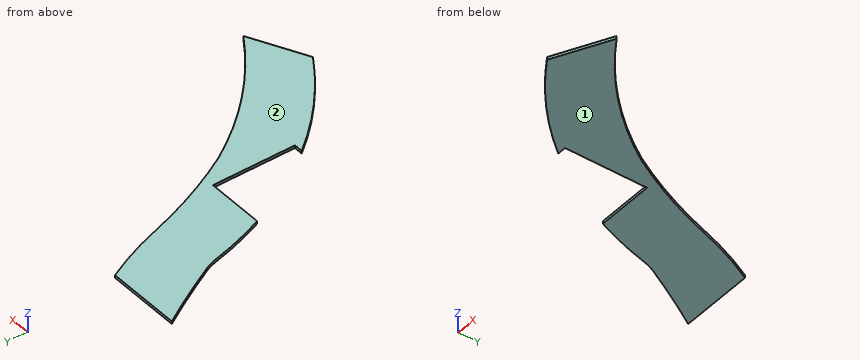
from build123d import *

# Parameters (mm, degrees)
SALIENTE_EXTRUIR1_DEPTH = 0.1


with BuildPart() as part:
    # Model → Saliente-Extruir1 (new body)
    with BuildSketch(Plane.XY):
        with BuildLine():
            Line((34.649371272, 11.960982991), (32.649371272, 10.960982991))
            ThreePointArc((32.649371272, 10.960982991), (30.912697203, 12.270631548), (29.428783982, 13.860982991))
            Line((29.428783982, 13.860982991), (29.750628728, 13.860982991))
            Line((29.750628728, 13.860982991), (29.750628728, 16.860982991))
            Line((29.750628728, 16.860982991), (27.658106466, 16.860982991))
            ThreePointArc((27.658106466, 16.860982991), (27.286967067, 17.858065763), (26.999339741, 18.882365051))
            ThreePointArc((26.999339741, 18.882365051), (26.927371, 19.119642667), (26.826595189, 19.346191565))
            ThreePointArc((26.826595189, 19.346191565), (26.1936862, 20.505212953), (25.516639133, 21.639017009))
            Line((25.516639133, 21.639017009), (28.203922027, 21.639017009))
            ThreePointArc((28.203922027, 21.639017009), (28.714965722, 20.556705993), (29.121100427, 19.430820834))
            ThreePointArc((29.121100427, 19.430820834), (29.792213257, 17.653647808), (30.650628728, 15.958991716))
            ThreePointArc((30.650628728, 15.958991716), (32.427042415, 13.736988846), (34.649371272, 11.960982991))
        make_face()
    extrude(amount=SALIENTE_EXTRUIR1_DEPTH)


solid = part.part
Design review of the part built by this model. Coordinates are the model's own, in mm. Face numbers are marked on the shaded views. Give positions to 0.01 mm unless a question says otherwise; leave off trailing zeros. Loops run counter-clockwise (first coordinate to the right, second up) from the corner with the lowest first, then second, coordinate; pieces in that order, holes last. Notation, with made-up numbers: M 69,-26 L 99,-26 A15 ccw 99,-4 Z; hole C 81.5,5 d4. An arc over 180 degrees is marked long. Answer as a JSON object with one key per item and string values.
Item 1: For P1, Ø4, axis at x = 32, y = 13.5, coming from the -Z side, flat-tipped, find the tip position at first contact; note if it passes through.
Output values:
{"P1": "stops at z = 0"}
Item 2: Mouldability with a two-part tool opening along Z and no side actions: class the marked faces 1 and 2 as pulls with the +Z half, pulls with the -Z half, needs draft (parallel to the pull), parting line crosses it, or undercut.
Output values:
{"face 1": "pulls with the -Z half", "face 2": "pulls with the +Z half"}
Item 3: We need section A-A (z = 0.05). State the section outline as (x, y) points, and give its area (3 significant figures).
Output values:
{"outline": "M 25.52,21.64 A34.31 cw 26.83,19.35 A2 cw 27,18.88 A12.89 ccw 27.66,16.86 L 29.75,16.86 L 29.75,13.86 L 29.43,13.86 A12.53 ccw 32.65,10.96 L 34.65,11.96 A12.83 cw 30.65,15.96 A17.63 cw 29.12,19.43 A12.61 ccw 28.2,21.64 Z", "area": "23.4 mm2"}
Item 4: We need section C-C (x = 32.25). State the section outline as (y, z) points, and give its area (3 significant figures).
Output values:
{"outline": "M 11.22,0 L 13.92,0 L 13.92,0.1 L 11.22,0.1 Z", "area": "0.270 mm2"}
Item 5: Wall thickness on line 1 along X through (y, z) = (11.5, 0.05); line 2 along Y through (x, z) = (31, 0.05); line 3 along X through (y, z) = (14.5, 0.05): over which ranges is each line inside the solid? List them lowest first.
Output values:
{"line 1": "x = 31.86 to 33.73", "line 2": "y = 12.19 to 15.43", "line 3": "x = 29.75 to 31.72"}
Item 6: We need section B-B (y = 15). State the section outline as (x, z) points, and give its area (3 significant figures).
Output values:
{"outline": "M 29.75,0 L 31.32,0 L 31.32,0.1 L 29.75,0.1 Z", "area": "0.157 mm2"}
